Study the drawing (mm; zero at the part's minimum x, y, z) and answer. A direction names the side the tool comes from. Coordinates: 2 decimals unless noted, no trailing zeros. Loops run counter-clockwise (first coordinate to the right, second up) from the corner with the lowest first, then second, coordinate; pieces in that order, holes last. Notation, with made-up numbers: (86, 61) -> (133, 61) arc R19 ccw to (133, 78) -> close; hole circle Ø7 at (-8, -31.5). An arc over 180 degrees is marked (long way). Answer as a JSON object with one key per item and string values. Group by question number.
Q1. Determine the mould class of the marked faces 1, 2 and 3 for opening direction X: released by +X, released by -X, zero draft, split by the parting line, or undercut.
Q2. The part is cut by section C-C on z = 4. Write down the section's boundary in (x, y), and give its area (3 significant figures).
Q3. For the marked faces 4 and 5, determine the directions among +Z, -Z, +X, -X, +Y, -Y from which every point of the face is accessible in a straight line to the end or side of a thin tool.
Q4. The part is cut by section A-A on x = 23. Write down the section's boundary in (y, z).
Q5. Straight lines are drawn through the part: line 1 along X through (y, z) = (17.5, 17.5); line 2 along Y through (x, z) = (122, 10.25); line 3 along X through (y, z) = (6, 18.5). For each, find the intervals that lie inside material, in ascending order. Write a range as [from, to].
Q6. The part is cut by section B-B on y = 69. Write down the section's boundary in (x, z).
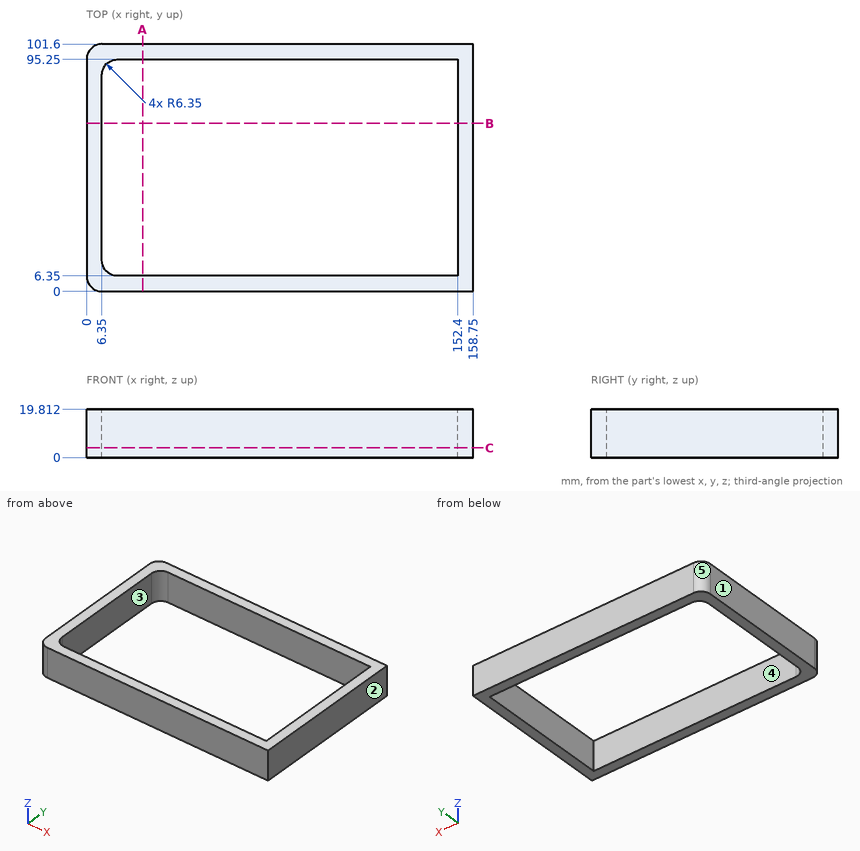
Final values:
{
 "1": {"face 1": "released by -X", "face 2": "released by +X", "face 3": "undercut"},
 "2": {"outline": "(0, 6.35) arc R6.35 ccw to (6.35, 0) -> (158.75, 0) -> (158.75, 101.6) -> (6.35, 101.6) arc R6.35 ccw to (0, 95.25) -> close; hole (6.35, 12.7) arc R6.35 ccw to (12.7, 6.35) -> (152.4, 6.35) -> (152.4, 95.25) -> (12.7, 95.25) arc R6.35 ccw to (6.35, 88.9) -> close", "area": "3,150 mm2"},
 "3": {"face 4": "+Z, -Z", "face 5": "+Z, -Z, -X, +Y"},
 "4": {"outline": "(0, 0) -> (6.35, 0) -> (6.35, 19.81) -> (0, 19.81) -> close; (95.25, 0) -> (101.6, 0) -> (101.6, 19.81) -> (95.25, 19.81) -> close"},
 "5": {"line 1": "x = [0, 6.35], [152.4, 158.75]", "line 2": "y = [0, 6.35], [95.25, 101.6]", "line 3": "x = [0.01, 158.75]"},
 "6": {"outline": "(0, 0) -> (6.35, 0) -> (6.35, 19.81) -> (0, 19.81) -> close; (152.4, 0) -> (158.75, 0) -> (158.75, 19.81) -> (152.4, 19.81) -> close"}
}
